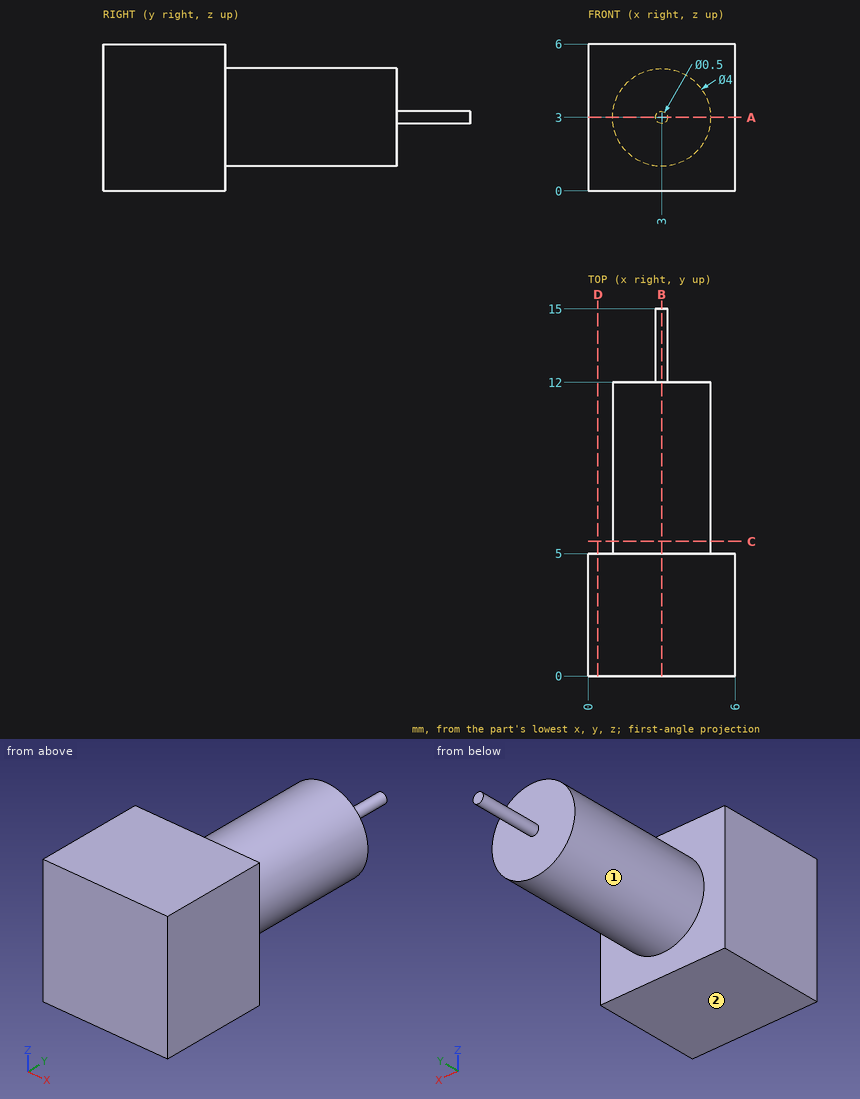
Can you work these out from the drawing? Everything is in mm from the part's minimum corner. A direction names the side the tool comes from. Give positions to 0.01 mm unless a question says otherwise; leave off trailing zeros. Order: outer loops, then holes, each group sorted by start corner. A loop starts at its lowest first (then second) coordinate and runs counter-clockwise, first axis right, second up. Notation, with made-up numbers: M 87,-10 L 138,-10 A18 cw 138,-1 Z; hole C 58.5,50 d7. An arc over 180 degrees is marked long. One line per question, with ' | ' between items.
1. I want a section at B-B (x = 3). List the corners of the cut face in (y, z) for me.
Results:
outline: M 0,0 L 5,0 L 5,1 L 12,1 L 12,2.75 L 15,2.75 L 15,3.25 L 12,3.25 L 12,5 L 5,5 L 5,6 L 0,6 Z
2. I'm going to push flat-ended pins straight in: pin 1 (1.5 mm diameter, centred on x = 4.5, y = 9, fed in from +Z); pin 2 (1.8 mm diameter, centred on x = 3, z = 1.5, fed in from +Y); pin 3 (2 mm diameter, centred on y = 8.5, z = 4.5, fed in from -X); pin 4 (3 mm diameter, centred on x = 2, z = 3.5, fed in from +Y). Where does each tip first touch, or does it pass through?
Results:
pin 1: z = 4.85 | pin 2: y = 12 | pin 3: x = 1.06 | pin 4: y = 15
3. I want a section at D-D (x = 0.4). List the corners of the cut face in (y, z) for me.
Results:
outline: M 0,0 L 5,0 L 5,6 L 0,6 Z
4. I want a section at A-A (z = 3). List the corners of the cut face in (x, y) for me, and give its area (3 significant figures).
Results:
outline: M 0,0 L 6,0 L 6,5 L 5,5 L 5,12 L 3.25,12 L 3.25,15 L 2.75,15 L 2.75,12 L 1,12 L 1,5 L 0,5 Z | area: 59.5 mm²
5. I want a section at C-C (y = 5.5). List the corners of the cut face in (x, z) for me.
Results:
outline: C 3,3 d4
6. If I drill on line 1 (Y direction, x = 4.2, z = 4.9); line 2 (Y direction, x = 3.1, z = 4.5); line 3 (Z direction, x = 3.1, y = 11), over which ranges is the centre line in solid material (lowest first)?
Results:
line 1: 0 to 5 | line 2: 0 to 12 | line 3: 1 to 5
7. For the marked faces 1 and 2, which set-ups out of +Z, -Z, +X, -X, +Y, -Y let a thin tool reach every point of the face, with its end or its side?
Results:
face 1: +Y | face 2: -Z, +X, -X, +Y, -Y
